The model under review builds one solid part; all positions refer to its coordinate system, in mm. A direction names the side the tool comes from. Round coordinates to 2 decimals unless told otherwise and drop trailing zeros. Order: outer loops, then holes, each group sorted by start corner. A loop starts at its lowest first (then second) coordinate and runs counter-clockwise, first axis right, second up. Notation, with made-up numbers: (81, -39) -> (122, -39) arc R23 cw to (122, -15) -> close; hole circle Ø2 at (42, -33). An arc over 180 degrees is marked (long way). Return JSON: item names as keys, results as strings. Group by question number.
from build123d import *

# Parameters (mm, degrees)
SKETCH2_R           = 1.7
BOSS_EXTRUDE1_DEPTH = 3.175
SKETCH3_W           = 60
SKETCH3_H           = 160.555920096
CUT_EXTRUDE1_DEPTH  = 4.175
SKETCH4_R           = 1.7
BOSS_EXTRUDE2_DEPTH = 19


with BuildPart() as part:
    # Sketch2 → Boss-Extrude1 (new body)
    with BuildSketch(Plane.XY):
        with BuildLine():
            Line((54.582717937, -59.58290593), (54.582717937, 171.394622999))
            ThreePointArc((54.582717937, 171.394622999), (24.582717937, 201.394622999), (-5.417282063, 171.394622999))
            Line((-5.417282063, 171.394622999), (-5.417282063, -59.58290593))
            ThreePointArc((-5.417282063, -59.58290593), (24.582717937, -89.58290593), (54.582717937, -59.58290593))
        make_face()
        with Locations((27.882717937, 197.940291196)):
            Circle(SKETCH2_R, mode=Mode.SUBTRACT)
        with Locations((-2.167282063, -59.58290593)):
            Circle(SKETCH2_R, mode=Mode.SUBTRACT)
        with Locations((5.667611541, -78.498012327)):
            Circle(SKETCH2_R, mode=Mode.SUBTRACT)
        with Locations((21.182717937, -86.115951364)):
            Circle(SKETCH2_R, mode=Mode.SUBTRACT)
        with Locations((51.332717937, 171.394622999)):
            Circle(SKETCH2_R, mode=Mode.SUBTRACT)
        with Locations((-2.167282063, 59.305858535)):
            Circle(SKETCH2_R, mode=Mode.SUBTRACT)
        with Locations((27.982717937, -86.115951364)):
            Circle(SKETCH2_R, mode=Mode.SUBTRACT)
        with Locations((-2.167282063, 171.394622999)):
            Circle(SKETCH2_R, mode=Mode.SUBTRACT)
        with Locations((51.332717937, 115.905858535)):
            Circle(SKETCH2_R, mode=Mode.SUBTRACT)
        with Locations((-2.167282063, 115.905858535)):
            Circle(SKETCH2_R, mode=Mode.SUBTRACT)
        with Locations((43.497824334, -78.498012327)):
            Circle(SKETCH2_R, mode=Mode.SUBTRACT)
        with Locations((51.332717937, -59.58290593)):
            Circle(SKETCH2_R, mode=Mode.SUBTRACT)
        with Locations((51.332717937, -34.094141465)):
            Circle(SKETCH2_R, mode=Mode.SUBTRACT)
        with Locations((-2.167282063, -34.094141465)):
            Circle(SKETCH2_R, mode=Mode.SUBTRACT)
        with Locations((51.332717937, -4.094141465)):
            Circle(SKETCH2_R, mode=Mode.SUBTRACT)
        with Locations((-2.167282063, -4.094141465)):
            Circle(SKETCH2_R, mode=Mode.SUBTRACT)
        with Locations((51.332717937, 25.905858535)):
            Circle(SKETCH2_R, mode=Mode.SUBTRACT)
        with Locations((-2.167282063, 25.905858535)):
            Circle(SKETCH2_R, mode=Mode.SUBTRACT)
        with Locations((21.282717937, 197.940291196)):
            Circle(SKETCH2_R, mode=Mode.SUBTRACT)
        with Locations((51.332717937, 52.505858535)):
            Circle(SKETCH2_R, mode=Mode.SUBTRACT)
        with Locations((51.332717937, 59.305858535)):
            Circle(SKETCH2_R, mode=Mode.SUBTRACT)
        with Locations((-2.167282063, 52.505858535)):
            Circle(SKETCH2_R, mode=Mode.SUBTRACT)
    extrude(amount=BOSS_EXTRUDE1_DEPTH)

    # Sketch3 → Cut-Extrude1 (cut, through all)
    with BuildSketch(Plane.XY.offset(3.175)):
        with Locations((24.582717937, -24.372101513)):
            Rectangle(SKETCH3_W, SKETCH3_H)
    extrude(amount=-CUT_EXTRUDE1_DEPTH, mode=Mode.SUBTRACT)

    # Sketch4 → Boss-Extrude2 (add)
    with BuildSketch(Plane.XY.offset(3.175)):
        with BuildLine():
            Line((48.082717937, 171.394622999), (48.082717937, 55.905858535))
            Line((48.082717937, 55.905858535), (54.582717937, 55.905858535))
            Line((54.582717937, 55.905858535), (54.582717937, 171.394622999))
            ThreePointArc((54.582717937, 171.394622999), (24.582717937, 201.394622999), (-5.417282063, 171.394622999))
            Line((-5.417282063, 171.394622999), (-5.417282063, 55.905858535))
            Line((-5.417282063, 55.905858535), (1.082717937, 55.905858535))
            Line((1.082717937, 55.905858535), (1.082717937, 171.394622999))
            ThreePointArc((1.082717937, 171.394622999), (24.582717937, 194.894622999), (48.082717937, 171.394622999))
        make_face()
        with Locations((-2.167282063, 115.905858535)):
            Circle(SKETCH4_R, mode=Mode.SUBTRACT)
        with Locations((-2.167282063, 59.305858535)):
            Circle(SKETCH4_R, mode=Mode.SUBTRACT)
        with Locations((51.332717937, 59.305858535)):
            Circle(SKETCH4_R, mode=Mode.SUBTRACT)
        with Locations((51.332717937, 115.905858535)):
            Circle(SKETCH4_R, mode=Mode.SUBTRACT)
        with Locations((51.332717937, 171.394622999)):
            Circle(SKETCH4_R, mode=Mode.SUBTRACT)
        with Locations((27.882717937, 197.940291196)):
            Circle(SKETCH4_R, mode=Mode.SUBTRACT)
        with Locations((21.282717937, 197.940291196)):
            Circle(SKETCH4_R, mode=Mode.SUBTRACT)
        with Locations((-2.167282063, 171.394622999)):
            Circle(SKETCH4_R, mode=Mode.SUBTRACT)
    extrude(amount=BOSS_EXTRUDE2_DEPTH)


solid = part.part
Item 1: The part is to be moulded in two halves that separate along X. For faces 3 (the face through (29.453, 197.289, 10.932)), 4 (the face through (25.242, 201.387, 10.932)), 5 (the face through (54.583, 113, 11)), say which applies: +X half, -X half, draft (parallel to the pull), parting line (faces both ways), or undercut.
Item 2: For faces 1 (the face through (24, 130, 0)), 2 (the face through (48.083, 114, 13)), list the 3-axis set-ups (+Z, -Z, +X, -X, +Y, -Y) from which the entire face can be reached by the end or side of a thin tool; tool diameter is ignored.
Item 3: Insertion check: pin 1 Ø4.5 at (x, y) = (27.88, 197.94) entering from -Z; pin 2 Ø5 at (x, y) = (7, 163.5) entering from +Z (3 decimals); pin 3 Ø10 at (x, z) = (44, 16) entering from +Y; pin 4 Ø2 at (y, z) = (185.5, 9) entering from -X. Each pin has a flat end and moves straight along its axis. Give the tip position at first contact, or say it passes through.
Item 4: Consider section B-B on z = 12.75. Give the number of separate pieces and of enclosed holes in the cut face, plus the area to 3 significant figures.
Item 5: Wall thickness on line 1 along X through (y, z) = (94.5, 21.5); line 2 along Y through (x, z) = (50.5, 17.5); line 3 along Z through (x, y) = (35, 182) (3 decimals): over which ranges is each line inside the solid? List them lowest first.
Item 6: Consider section A-A on x = 51. State the section outline as (y, z) points (1 decimal), plus the area to 3 significant figures.
Item 7: Consider section D-D on x = 15.5. State the section outline as (y, z) points (3 decimals).
Item 8: Consider section C-C on y = 88. State the section outline as (x, z) points (3 decimals), plus the area to 4 significant figures.
Values:
{
 "1": {"face 3": "undercut", "face 4": "parting line", "face 5": "+X half"},
 "2": {"face 1": "-Z, +X, -X, +Y, -Y", "face 2": "+Z, -Y"},
 "3": {"pin 1": "z = 0", "pin 2": "z = 3.175", "pin 3": "y = 197.7", "pin 4": "x = -2.4"},
 "4": {"separate pieces": "1", "enclosed holes": "8", "area": "1,970 mm^2"},
 "5": {"line 1": "-5.42 to 1.08, 48.08 to 54.58", "line 2": "55.91 to 57.82, 60.79 to 114.42, 117.39 to 169.91, 172.88 to 186.5", "line 3": "0 to 3.175"},
 "6": {"outline": "(55.9, 0) -> (57.6, 0) -> (57.6, 22.2) -> (55.9, 22.2) -> close; (61, 0) -> (114.2, 0) -> (114.2, 22.2) -> (61, 22.2) -> close; (117.6, 0) -> (169.7, 0) -> (169.7, 22.2) -> (117.6, 22.2) -> close; (173.1, 0) -> (185.6, 0) -> (185.6, 22.2) -> (173.1, 22.2) -> close", "area": "2,650 mm^2"},
 "7": {"outline": "(55.906, 0) -> (199.987, 0) -> (199.987, 22.175) -> (193.068, 22.175) -> (193.068, 3.175) -> (55.906, 3.175) -> close"},
 "8": {"outline": "(-5.417, 0) -> (54.583, 0) -> (54.583, 22.175) -> (48.083, 22.175) -> (48.083, 3.175) -> (1.083, 3.175) -> (1.083, 22.175) -> (-5.417, 22.175) -> close", "area": "437.5 mm^2"}
}
